from build123d import *

# Parameters (mm, degrees)
SKETCH023_R     = 1.640991
SKETCH023_R_2   = 1.667929
PAD017_DEPTH    = 2
SKETCH024_W     = 1.10811
SKETCH024_H     = 5.765145
PAD018_DEPTH    = 4.6
CHAMFER004_SIZE = 0.5


with BuildPart() as part:
    # Sketch023 → Pad017 (new body)
    with BuildSketch(Plane.XY):
        with BuildLine():
            ThreePointArc((59.303531, 33.743852), (55.880409, 37.166974), (52.457287, 33.743852))
            Line((52.457287, 33.743852), (52.303531, 20.99579))
            ThreePointArc((52.303531, 20.99579), (55.803531, 17.49579), (59.303531, 20.99579))
            Line((59.303531, 33.743852), (59.303531, 20.99579))
        make_face()
        with Locations((55.880409, 33.743852)):
            Circle(SKETCH023_R, mode=Mode.SUBTRACT)
        with Locations((55.803531, 20.99579)):
            Circle(SKETCH023_R_2, mode=Mode.SUBTRACT)
    extrude(amount=PAD017_DEPTH)

    # Sketch024 → Pad018 (join)
    with BuildSketch(Plane.XY):
        with Locations((54.015807, 27.08314)):
            Rectangle(SKETCH024_W, SKETCH024_H)
        with Locations((57.761141, 27.08314)):
            Rectangle(SKETCH024_W, SKETCH024_H)
    extrude(amount=PAD018_DEPTH)

    # Chamfer004
    chamfer004_edges = [part.edges().sort_by_distance(p)[0] for p in [
        (54.135602, 20.99579, 0),
        (54.239418, 33.743852, 0),
    ]]
    chamfer(chamfer004_edges, length=CHAMFER004_SIZE)


solid = part.part
The model under review builds one solid part; all positions refer to its coordinate system, in mm. A direction names the side the tool comes from. Coordinates: 2 decimals unless noted, no trailing zeros. Loops run counter-clockwise (first coordinate to the right, second up) from the corner with the lowest first, then second, coordinate; pieces in that order, holes last. Notation, with made-up numbers: M 52.25,-8 L 81.25,-8 A12 ccw 81.25,0 Z; hole C 33.25,45 d8. An arc over 180 degrees is marked long. Put each result on its own line as item: value. Start each with the question number.
Q1. Clearance check with flat-ended pins moving along their axes: pin 1 (1.3 mm diameter, centred on y = 26.5, z = 3.5, fed in from -X); pin 2 (1.5 mm diameter, centred on x = 57, y = 20.5, fed in from +Z); pin 3 (0.9 mm diameter, centred on x = 57.5, z = 3.5, fed in from -Y). State where each tip first meets the part, or that it passes through.
Q2. Add section B-B (z = 1.3). Write out the cut boundary in (x, y).
Q3. Add section D-D (x = 57). Count the separate pieces of the cut face and the enclosed holes in it, and give its area (3 significant figures).
Q4. Add section C-C (y = 25.5). Write out the cut boundary in (x, z).
Q5. Add section A-A (z = 3.5). Write out the cut boundary in (x, y).
Q6. Wall thickness on line 1 (X direction, y = 26.5, z = 2.5); line 2 (Y direction, x = 56, z = 0.7); line 3 (Y direction, x = 56.75, z = 0.35): over which ranges is each line inside the solid? List them lowest first.
Q7. The part is to be moulded in two halves that separate along X. For faces 4 (the cylindrical face through (55.727, 17.497, 0.986)), 5 (the flat face through (54.57, 27, 3)), 6 (the flat face through (54, 29.966, 3)), say which applies: +X half, -X half, draft (parallel to the pull), parting line (faces both ways), or undercut.
Q8. For faces 1 (the flat face through (58.315, 27, 3)), 2 (the flat face through (54, 24.201, 3)), 3 (the flat face through (58, 29.966, 3)), list the 3-axis set-ups (+Z, -Z, +X, -X, +Y, -Y) from which the entire face can be reached by the end or side of a thin tool; tool diameter is ignored.
Answers:
1. pin 1: stops at x = 53.46
1. pin 2: stops at z = 2
1. pin 3: stops at y = 24.2
2. outline: M 52.3,21 A3.5 ccw 59.3,21 L 59.3,33.74 A3.42 ccw 52.46,33.74 Z; hole C 55.8,21 d3.34; hole C 55.88,33.74 d3.28
3. separate pieces: 3
3. enclosed holes: 0
3. area: 28.4 mm^2
4. outline: M 52.36,0 L 59.3,0 L 59.3,2 L 58.32,2 L 58.32,4.6 L 57.21,4.6 L 57.21,2 L 54.57,2 L 54.57,4.6 L 53.46,4.6 L 53.46,2 L 52.36,2 Z
5. outline: M 53.46,24.2 L 54.57,24.2 L 54.57,29.97 L 53.46,29.97 Z; M 57.21,24.2 L 58.32,24.2 L 58.32,29.97 L 57.21,29.97 Z
6. line 1: x = 53.46 to 54.57, 57.21 to 58.32
6. line 2: y = 17.5 to 19.34, 22.65 to 32.11, 35.38 to 37.16
6. line 3: y = 17.63 to 19.44, 22.55 to 32.18, 35.31 to 37.05
7. face 4: parting line
7. face 5: undercut
7. face 6: draft
8. face 1: +Z, +X, +Y, -Y
8. face 2: +Z, +X, -X, -Y
8. face 3: +Z, +X, -X, +Y
